Answer from the drawing. Dimensions are ordinates in mm from the lowest x, y and z of the part. A direction names the side the tool comes from. Give positions to 0.01 mm unless a question says otherwise; leave off trailing zeros. Loops run counter-clockwise (first coordinate to the right, second up) from the corner with the lowest first, then second, coordinate; pieces in that order, holes last.
Item 1: The mould has two halves that part along Y. Classify the marked faces 4, 5 and 6: pulls with the +Y half, pulls with the -Y half, needs draft (parallel to the pull), parting line crosses it, or undercut.
Item 2: A tool of negligible diameter and unlimited length cuts with its end or side. For the marked faces 1, 2 and 3, from which of +Z, -Z, +X, -X, +Y, -Y can it reach the whole face along a straight path? Write none if from no direction.
Item 3: Section A-A, the plane z = 7 is taken. Give the vertices of the cut face in (x, y), and give its area (3 significant figures).
Item 4: Consider line 1 along X through (y, z) = (8, 4.5); line 2 along Y through (x, z) = (5, 6); line 3 along Y through (x, z) = (5, 3.5). Determine where each line is inside the solid, lowest interval first.
Item 5: Section C-C, the plane y = 7 is taken. Give the vertices of the cut face in (x, z).
Item 6: Section B-B, the plane z = 9 is taken. Give the vertices of the cut face in (x, y).
Item 7: Each of these flat-tipped pins is pushed along its axis until it touches: pin 1 Ø2 at (x, z) = (5.5, 5) entering from -Y; pin 2 Ø3 at (y, z) = (3, 7) entering from -X; pin 3 Ø1 at (x, z) = (7, 4.5) entering from -Y; pin 4 Ø5.5 at (x, y) = (5, 15) entering from +Z. Where does it stop, or does it pass through?
Item 8: Section D-D, the plane y = 15.5 is taken. Give the vertices of the cut face in (x, z), and give its area (3 significant figures).
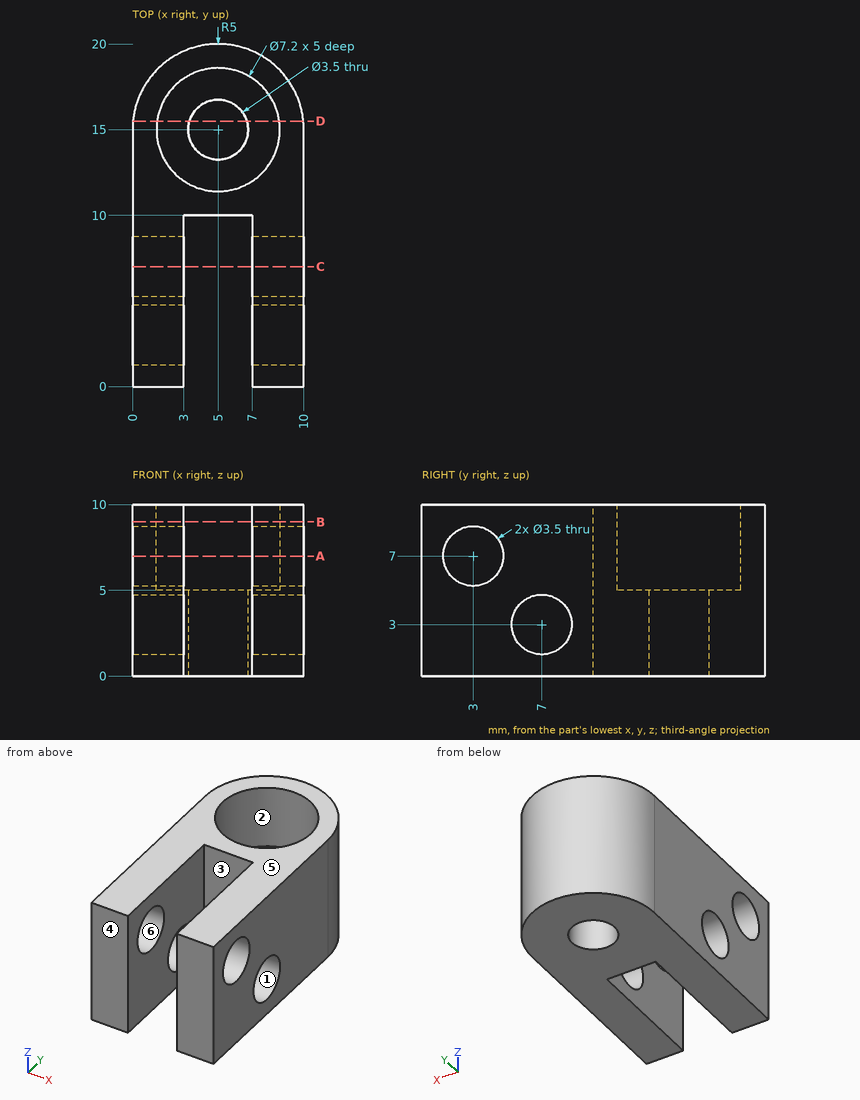
Worked answers:
1. face 4: pulls with the -Y half
1. face 5: needs draft
1. face 6: undercut
2. face 1: +X, -X
2. face 2: +Z
2. face 3: +Z, -Z, -Y
3. outline: (0, 0) - (3, 0) - (3, 1.25) - (0, 1.25) - close; (0, 4.75) - (3, 4.75) - (3, 10) - (7, 10) - (7, 4.75) - (10, 4.75) - (10, 15) arc R5 ccw to (0, 15) - close; (7, 0) - (10, 0) - (10, 1.25) - (7, 1.25) - close; hole circle Ø7.2 at (5, 15)
3. area: 87.6 mm2
4. line 1: x = 0 to 3, 7 to 10
4. line 2: y = 10 to 11.4, 18.6 to 20
4. line 3: y = 10 to 13.25, 16.75 to 20
5. outline: (0, 0) - (3, 0) - (3, 1.25) - (0, 1.25) - close; (0, 4.75) - (3, 4.75) - (3, 10) - (0, 10) - close; (7, 0) - (10, 0) - (10, 1.25) - (7, 1.25) - close; (7, 4.75) - (10, 4.75) - (10, 10) - (7, 10) - close
6. outline: (0, 0) - (3, 0) - (3, 10) - (7, 10) - (7, 0) - (10, 0) - (10, 15) arc R5 ccw to (0, 15) - close; hole circle Ø7.2 at (5, 15)
7. pin 1: stops at y = 10
7. pin 2: passes through
7. pin 3: stops at y = 0
7. pin 4: stops at z = 5
8. outline: (0.03, 0) - (3.32, 0) - (3.32, 5) - (1.43, 5) - (1.43, 10) - (0.03, 10) - close; (6.68, 0) - (9.97, 0) - (9.97, 10) - (8.57, 10) - (8.57, 5) - (6.68, 5) - close
8. area: 47.1 mm2
